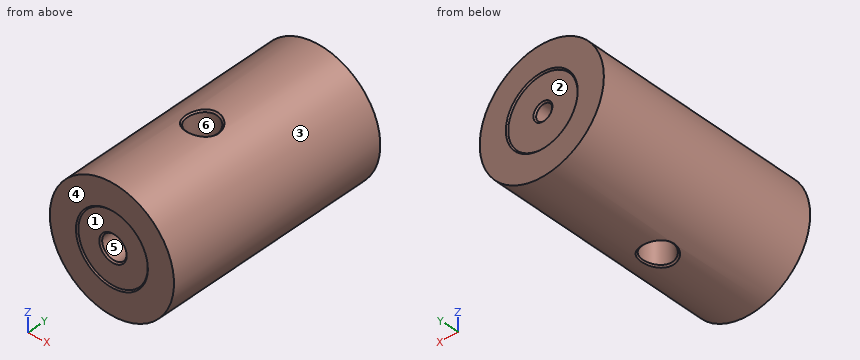
Autodesk Inventor part; units mm, degrees
ref_plane "YZ Plane" through (0, 0, 0) normal (1, 0, 0) x (0, 1, 0)
ref_plane "XZ Plane" through (0, 0, 0) normal (0, 1, 0) x (-1, 0, 0)
ref_plane "XY Plane" through (0, 0, 0) normal (0, 0, 1) x (1, 0, 0)
sketch "Sketch1" plane through (0, 0, 0) normal (0, 1, 0) x (-1, 0, 0)
  circle A0 centre (0, 0) radius 12.5
  dimension "d0" = 25
extrude "Extrusion1" add sketch "Sketch1" along normal blind 45.7
hole "ReliefTop" at (0, 45.7, 0) direction (0, -1, 0) diameter 13.97 depth 0.254 countersink diameter 14.478 countersink angle 90
hole "ReliefBottom" at (0, 0, 0) direction (0, 1, 0) diameter 13.97 depth 0.254 countersink diameter 14.478 countersink angle 90
hole "MountBottomM6" at (0, 0.254, 0) direction (0, 1, 0) diameter 4.917 depth 7.366 tip angle 118 countersink diameter 5.508 countersink angle 90
hole "MountTopM4" at (0, 45.446, 0) direction (0, -1, 0) diameter 3.242 depth 14.478 tip angle 118 countersink diameter 3.808 countersink angle 90
sketch "Sketch2" plane through (0, 0, 0) normal (0, 0, 1) x (1, 0, 0)
  circle A0 centre (0, 20) radius 3
  line L0 (-12.5, 0) -> (12.5, 0)
  line L1 (0, -4.6) -> (0, 27.6)
  point P0 (0, 0)
  dimension "d49" = 6
  dimension "d50" = 20
extrude "Extrusion2" cut sketch "Sketch2" along normal through all both and the other way through all
chamfer "Chamfer1" distance 0.313 angle 45 2 edges at (-3, 19.9998, 12.1347) (-3, 19.9998, -12.1347)
equation "\"d1\" = height"
equation "\"d5\" = reliefMinor"
equation "\"d7\" = reliefMajor"
equation "\"d10\" = reliefDepth"
equation "\"d14\" = reliefMinor"
equation "\"d16\" = reliefMajor"
equation "\"d19\" = reliefDepth"
equation "\"d25\" = chamferM6"
equation "\"d28\" = depthM6"
equation "\"d40\" = chamferM4"
equation "\"d43\" = depthM4"
equation "\"reliefDepth\" = 0.254"
equation "\"reliefMinor\" = 13.97"
equation "\"reliefMajor\" = 14.478"
equation "\"chamferM6\" = 5.508"
equation "\"chamferM4\" = 3.808"
equation "\"depthM6\" = 7.366"
equation "\"depthM4\" = 14.478"
equation "\"height\" = 45.7"
properties part number "PLS-P642H0457A00_M" material "Stainless Steel"
Verification items for the finished model (mm, model axes). Face numbers are marked on the shaded views. A direction names the side the tool comes from. Coordinates: 2 decimals unless noted, no trailing zeros. Order: outer loops, then holes, each group sorted by start corner. A loop starts at its lowest first (then second) coordinate and runs counter-clockwise, first axis right, second up. Notation, with made-up numbers: (23.5, 33.5) -> (41.5, 33.5) arc R27 ccw to (41.5, 67.5) -> close; hole circle Ø7 at (7, 66). An arc over 180 degrees is marked (long way). Put each result on its own line as item: value. Start each with the question number.
1) Cross-section at A-A (z = 10). Enter the section's corners in (x, y).
2) Cross-section at C-C (y = 12.5). Enter the section's corners in (x, z), plus the area to 3 significant figures.
3) Material ranges on L1, parallel to Y at x = 0, z = -3.25; L2, parallel to Z at x = 0, y = 5.5; L3, parallel to Z at x = 0, y = 39, recorded low to high.
4) Tool access check on the marked faces 5 and 6. Record the directions out of +Z, -Z, +X, -X, +Y, -Y that give a thin tool (end or side, any length) a straight path to the whole face; none if there is none.
5) Cross-section at B-B (y = 3.5). Enter the section's corners in (x, z), plus the area to 3 significant figures.
6) Release check for a two-part mould opening along X. For the marked faces 1, 2, 3 and 4 record: pulls with the +X half, pulls with the -X half, needs draft (parallel to the pull), parting line crosses it, or undercut.
7) Go/stop test with flat-tipped pins: pin 1 (8 mm diameter, centred on x = 4.5, z = -4, fed in from +Y); pin 2 (6 mm diameter, centred on x = 0.5, z = -1.5, fed in from -Y); pin 3 (6 mm diameter, centred on y = 23, z = 5.5, fed in from +X); pin 4 (3.5 mm diameter, centred on x = 0, z = 0, fed in from -Y). Record where each tip stops, or that it passes through.
8) Cross-section at D-D (x = 7.75). Enter the section's corners in (y, z), plus the area to 3 significant figures.
Geometry check:
1. outline: (-7.5, 0) -> (7.5, 0) -> (7.5, 45.7) -> (-7.5, 45.7) -> close; hole circle Ø6 at (0, 20)
2. outline: circle Ø25 at (0, 0)
2. area: 491 mm^2
3. L1: y = 0.25 to 17, 23 to 45.45
3. L2: z = -12.5 to -2.46, 2.46 to 12.5
3. L3: z = -12.5 to -1.62, 1.62 to 12.5
4. face 5: -Y
4. face 6: +Z, -Z
5. outline: circle Ø25 at (0, 0); hole circle Ø4.92 at (0, 0)
5. area: 472 mm^2
6. face 1: undercut
6. face 2: undercut
6. face 3: parting line crosses it
6. face 4: needs draft
7. pin 1: stops at y = 45.7
7. pin 2: stops at y = 0.25
7. pin 3: stops at x = 12.25
7. pin 4: stops at y = 8.05
8. outline: (0, -9.81) -> (45.7, -9.81) -> (45.7, 9.81) -> (0, 9.81) -> close
8. area: 896 mm^2
